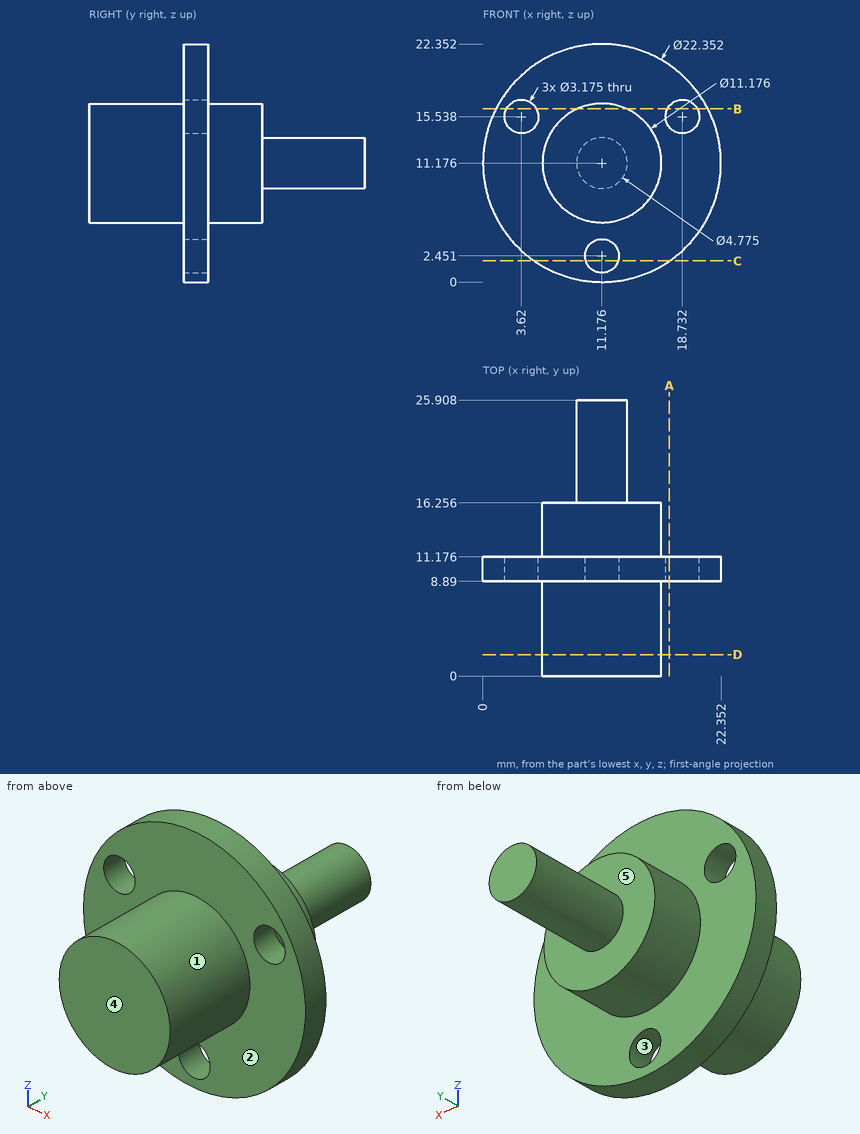
Here's the drawing with two shaded views (mm, measured from the low corner). I have some questions. A direction names the side the tool comes from. Give positions to 0.01 mm unless a question says otherwise; leave off trailing zeros. Order: outer loops, then holes, each group sorted by start corner. A loop starts at its lowest first (then second) coordinate and runs counter-clockwise, first axis right, second up. Notation, with made-up numbers: M -8.75,48.5 L 21.25,48.5 A20 ccw 21.25,79.5 Z; hole C 18.5,-5 d2. An arc over 180 degrees is marked long. Answer as a JSON object with one key per item and string values. Group by question number.
1) Suppose I cut it at D-D, the plane y = 2. Write out the boundary of the cut face in (x, z).
2) Suppose I cut it at A-A, the plane x = 17.5. Write out the boundary of the cut face in (y, z).
3) Suppose I cut it at B-B, the plane z = 16.25. Write out the boundary of the cut face in (x, y) (1 decimal).
4) Please list where these lines run through material, in increasing order: L1, parallel to X at y = 9, z = 15.75 (1 decimal); L2, parallel to Y at x = 2.5, z = 13.25; L3, parallel to Y at x = 10, z = 13.75. Write a range as [from, to].
5) On a 3-axis mill with a long thin cutter (end or side, diameter ignored), from which of +Z, -Z, +X, -X, +Y, -Y can I reach the whole of each face in a straight line? I mean the marked faces 4 and 5. Say none if no direction works.
6) We'd pull the mould along X, two halves only. Please class the marked faces 1, 2 and 3: pulls with the +X half, pulls with the -X half, needs draft (parallel to the pull), parting line crosses it, or undercut.
7) I'm going to push flat-ended pins straight in: pin 1 Ø2.5 at (x, z) = (3.62, 15.54) entering from +Y; pin 2 Ø5 at (x, z) = (17.5, 18) entering from +Y; pin 3 Ø3 at (x, y) = (16, 16) entering from +Z; pin 4 Ø3 at (y, z) = (6.5, 15.5) entering from +X. Where does each tip first touch, or does it pass through?
8) Suppose I cut it at C-C, the plane z = 2. Write out the boundary of the cut face in (x, y).
Results found:
{
 "1": {"outline": "C 11.18,11.18 d11.18"},
 "2": {"outline": "M 8.89,1.96 L 11.18,1.96 L 11.18,14.54 L 8.89,14.54 Z; M 8.89,16.54 L 11.18,16.54 L 11.18,20.39 L 8.89,20.39 Z"},
 "3": {"outline": "M 1.2,8.9 L 2.2,8.9 L 2.2,11.2 L 1.2,11.2 Z; M 5,8.9 L 8.8,8.9 L 8.8,0 L 13.5,0 L 13.5,8.9 L 17.3,8.9 L 17.3,11.2 L 13.5,11.2 L 13.5,16.3 L 8.8,16.3 L 8.8,11.2 L 5,11.2 Z; M 20.2,8.9 L 21.1,8.9 L 21.1,11.2 L 20.2,11.2 Z"},
 "4": {"L1": "[1, 2], [5.2, 17.2], [20.3, 21.4]", "L2": "[8.89, 11.18]", "L3": "[0, 16.26]"},
 "5": {"face 4": "+Z, -Z, +X, -X, -Y", "face 5": "+Y"},
 "6": {"face 1": "parting line crosses it", "face 2": "needs draft", "face 3": "undercut"},
 "7": {"pin 1": "through", "pin 2": "y = 11.18", "pin 3": "z = 15.67", "pin 4": "x = 16"},
 "8": {"outline": "M 4.8,8.89 L 9.65,8.89 L 9.65,11.18 L 4.8,11.18 Z; M 12.7,8.89 L 17.56,8.89 L 17.56,11.18 L 12.7,11.18 Z"}
}
